from build123d import *

# Parameters (mm, degrees)
BOSS_EXTRUDE1_DEPTH = 20
SKETCH5_W           = 15
SKETCH5_H           = 15
CUT_EXTRUDE1_DEPTH  = 40
SKETCH6_R           = 3
CUT_EXTRUDE2_DEPTH  = 34
FILLET1_R           = 15
FILLET2_R           = 15
FILLET3_R           = 25
FILLET4_R           = 10
CUT_EXTRUDE3_DEPTH  = 34
FILLET5_R           = 10


# Some blends are built 0.0001 mm under size
with BuildPart() as part:
    # Sketch3 → Boss-Extrude1 (new body)
    with BuildSketch(Plane(origin=(0, 0, 0), x_dir=(1, 0, 0), z_dir=(0, 1, 0))):
        Polygon((0, 0), (30.5, 0), (30.5, 60), (29.894285691, 64.601573483), (8.489458289, 90.110853439), (0.829013858, 83.682977342), (19.5341333, 61.391084047), (19.5341333, 31.391084047), (0, 15), align=None)
    extrude(amount=BOSS_EXTRUDE1_DEPTH)

    # Sketch5 → Cut-Extrude1 (cut)
    with BuildSketch(Plane(origin=(30.5, 0, 0), x_dir=(0, 0, -1), z_dir=(1, 0, 0))):
        with Locations((7.5, 7.5)):
            Rectangle(SKETCH5_W, SKETCH5_H)
    extrude(amount=-CUT_EXTRUDE1_DEPTH, mode=Mode.SUBTRACT)

    # Sketch6 → Cut-Extrude2 (cut)
    with BuildSketch(Plane(origin=(0, 20, 0), x_dir=(1, 0, 0), z_dir=(0, 1, 0))):
        with Locations(Location((15.25, 7.5, 0), (0, 0, 270))):
            Circle(SKETCH6_R)
    extrude(amount=-CUT_EXTRUDE2_DEPTH, mode=Mode.SUBTRACT)

    # Fillet1
    fillet1_edges = [part.edges().sort_by_distance(p)[0] for p in [
        (0, 17.5, 0),
        (30.5, 17.5, 0),
    ]]
    fillet(fillet1_edges, radius=FILLET1_R - 0.0001)  # a hair under: the kernel refuses the full size

    # Fillet2
    fillet2_edges = [part.edges().sort_by_distance(p)[0] for p in [
        (30.5, 7.5, -15),
    ]]
    fillet(fillet2_edges, radius=FILLET2_R)

    # Fillet3
    # the kernel refuses this fillet: 25 mm, written as the material it takes off along each edge
    with BuildSketch(Plane(origin=(29.894285691, -17.425359882, -64.601573483), x_dir=(-0.64278760968654, 0, -0.7660444431189775), z_dir=(0, 1, 0))) as fillet3_piece_1:
        with BuildLine():
            CenterArc((6.970143953, 25), FILLET3_R, 244.190525193, 25.809474807)
            Line((-3.914355449, 2.49383034), (-4.132045437, 2.043706946))
            ThreePointArc((-4.132045437, 2.043706946), (-2.225836026, 0.825224861), (-0.268658302, -0.421690309))
            Line((-0.268658302, -0.421690309), (0, -0.5))
            Line((0, -0.5), (6.970143953, -0.5))
            Line((6.970143953, -0.5), (6.970143953, 0))
        make_face()
    extrude(amount=54.850719763, mode=Mode.SUBTRACT)

    # Fillet4
    fillet4_edges = [part.edges().sort_by_distance(p)[0] for p in [
        (19.5341333, 10, -61.391084047),
    ]]
    fillet(fillet4_edges, radius=FILLET4_R)

    # Sketch7 → Cut-Extrude3 (cut)
    with BuildSketch(Plane(origin=(49.352752173, 0, -41.411876146), x_dir=(-0.6427876096865405, 0, -0.7660444431189772), z_dir=(0.7660444431189772, 0, -0.6427876096865404))):
        Polygon((56.07199994, 20), (63.57199994, 20), (63.57199994, 12.5), align=None)
    extrude(amount=-CUT_EXTRUDE3_DEPTH, mode=Mode.SUBTRACT)

    # Fillet5
    fillet5_edges = [part.edges().sort_by_distance(p)[0] for p in [
        (30.5, 10, -60),
    ]]
    fillet(fillet5_edges, radius=FILLET5_R)


solid = part.part
Part model, mm, in its own coordinate system. A direction names the side the tool comes from. Coordinates: 2 decimals unless noted, no trailing zeros. Loops run counter-clockwise (first coordinate to the right, second up) from the corner with the lowest first, then second, coordinate; pieces in that order, holes last. Notation, with made-up numbers: (-8, 36.25) -> (-2, 36.25) arc R31 ccw to (-2, 68.25) -> close; hole circle Ø9 at (1.25, 60). An arc over 180 degrees is marked (long way). Use a Markdown table: item, result. Add a question column.
Item 1: Band-saw the part on D-D on x = 29. Write the cut outline in (y, z), plus the area to 3 significant figures.
Item 2: Band-saw the part on B-B on z = -7.5. Write the cut outline in (x, y), plus the area to 3 significant figures.
Item 3: Probe probe 1 along X at (y, z) = (6.25, -41.5); probe 2 along Z at (x, y) = (9.5, 2.25); probe 3 along X at (y, z) = (18.9, -7.5). List the from-to ranges inside material, lowest first.
Item 4: Flat gauge pins, fed straight in: P1, Ø2, axis at x = 22, y = 5, coming from the -Z side; P2, Ø10, axis at x = 24, y = 12.5, coming from the -Z side; P3, Ø3, axis at y = 7.5, z = -16.5, coming from the +X side; P4, Ø15, axis at x = 11, z = -14, coming from the -Y side. Where does each tip first touch, or does it go through?
Item 5: Band-saw the part on A-A on y = 4.25. Write the cut outline in (x, z), plus the area to 3 significant figures.
Item 6: Pull direction Z, two halves, no side cores. Call faces 1 (the cylindrical face through (30.376, 10.14, -60.166)), 2 (the cylindrical face through (4.51, 17.54, -4.28)), 3 (the cylindrical face through (12.588, 17.535, -6.116)): +Z half, -Z half, draft (parallel to the pull), parting line (faces both ways), or undercut.
Item 7: Which spindle directions (+Z, -Z, +X, -X, +Y, -Y) get a long thin tool onto all of the face, cutting with end or side? Do faces 4 (the flat face through (4.71, 6.16, -86.94)), 5 (the flat face through (19.534, 10, -45)), 6 (the flat face through (8, 7, -15)), 7 (the cylindrical face through (26.22, 7.6, -19.51)). Say none if no direction does.
Item 8: Band-saw the part on C-C on z = -40. Write the cut outline in (x, y), plus the area to 3 significant figures.
Geometry says:
| question | item | result |
|---|---|---|
| 1 | outline | (0, -64.26) -> (20, -64.26) -> (20, -8.46) -> (15, -8.46) -> (15, -23.46) -> (0, -23.46) -> close |
| 1 | area | 891 mm² |
| 2 | outline | (2.01, 15) -> (12.25, 15) -> (12.25, 20) -> (2.01, 20) -> close; (18.25, 15) -> (28.49, 15) -> (28.49, 20) -> (18.25, 20) -> close |
| 2 | area | 102 mm² |
| 3 | probe 1 | 19.53 to 30.5 |
| 3 | probe 2 | -88.91 to -73.35, -22.97 to -15 |
| 3 | probe 3 | 2.01 to 12.25, 18.25 to 28.49 |
| 4 | P1 | z = -75.2 |
| 4 | P2 | z = -77.58 |
| 4 | P3 | x = 24.5 |
| 4 | P4 | y = 0 |
| 5 | outline | (0, -15) -> (19.53, -31.39) -> (19.53, -57.75) arc R10 cw to (17.19, -64.18) -> (0.83, -83.68) -> (8.49, -90.11) -> (25.41, -69.94) arc R25 ccw to (29.99, -61.74) arc R10 ccw to (30.5, -58.59) -> (30.5, -30) arc R15 ccw to (15.5, -15) -> close |
| 5 | area | 947 mm² |
| 6 | face 1 | -Z half |
| 6 | face 2 | +Z half |
| 6 | face 3 | undercut |
| 7 | face 4 | -Z, -X, +Y, -Y |
| 7 | face 5 | -X, +Y, -Y |
| 7 | face 6 | +Z, +X, -X, -Y |
| 7 | face 7 | +Z, +X, -Y |
| 8 | outline | (19.53, 0) -> (30.5, 0) -> (30.5, 20) -> (19.53, 20) -> close |
| 8 | area | 219 mm² |
